The model under review builds one solid part; all positions refer to its coordinate system, in mm. Face numbers are marked on the shaded views. A direction names the side the tool comes from. Coordinates: 2 decimals unless noted, no trailing zeros. Write each loop counter-clockwise with the first axis right and the second up, starting at its lowest first coordinate (ties: lowest second). Pieces come first, ordered by that corner, then holes. Notation, with made-up numbers: (-37.5, -25) - (1.5, -25) arc R19 cw to (1.5, -21) - close; hole circle Ø8 at (79, -20). An arc over 180 degrees is marked (long way). Put each result on its own line as item: value.
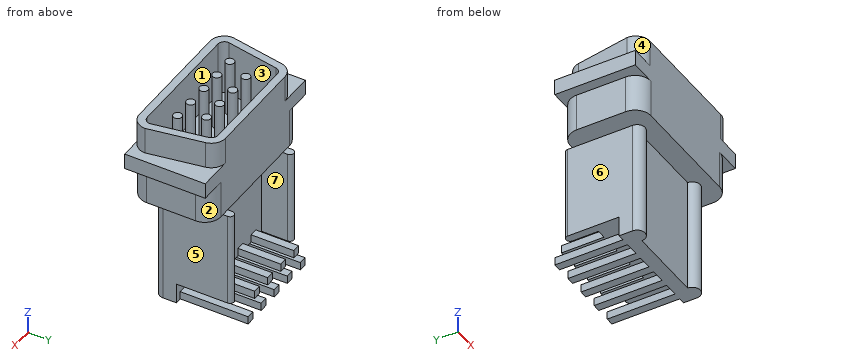
from build123d import *

# Parameters (mm, degrees)
SKETCH_1_W          = 21.2
SKETCH_1_H          = 10.2
EXTRUDE_1_DEPTH     = 2
EXTRUDE_2_DEPTH     = 3.4
EXTRUDE_3_DEPTH     = 4.8
EXTRUDE_4_DEPTH     = 12
EXTRUDE_5_DEPTH     = 2.6
SKETCH_6_R          = 0.545
CUT_EXTRUDE_1_DEPTH = 7
SKETCH_7_W          = 1
SKETCH_7_H          = 1
EXTRUDE_6_DEPTH     = 8.6
SKETCH_8_W          = 1
SKETCH_8_H          = 1
EXTRUDE_7_DEPTH     = 5.4


with BuildPart() as part:
    # Эскиз1 → Бобышка-Вытянуть1 (new body)
    with BuildSketch(Plane.XY):
        Rectangle(SKETCH_1_W, SKETCH_1_H)
    extrude(amount=EXTRUDE_1_DEPTH)

    # Эскиз2 → Бобышка-Вытянуть2 (add)
    with BuildSketch(Plane.XY.offset(2)):
        with BuildLine():
            Line((-6.3, 5.1), (6.3, 5.1))
            ThreePointArc((6.3, 5.1), (7.4561981, 4.679567307), (8.072281221, 3.614673282))
            Line((8.072281221, 3.614673282), (9.3, -3.3))
            ThreePointArc((9.3, -3.3), (8.772792206, -4.572792206), (7.5, -5.1))
            Line((7.5, -5.1), (-7.5, -5.1))
            ThreePointArc((-7.5, -5.1), (-8.772792206, -4.572792206), (-9.3, -3.3))
            Line((-9.3, -3.3), (-8.072281221, 3.614673282))
            ThreePointArc((-8.072281221, 3.614673282), (-7.4561981, 4.679567307), (-6.3, 5.1))
        make_face()
    extrude(amount=EXTRUDE_2_DEPTH)

    # Эскиз3 → Бобышка-Вытянуть3 (add)
    with BuildSketch(Plane(origin=(0, 0, 0), x_dir=(-1, 0, 0), z_dir=(0, 0, -1))):
        with BuildLine():
            Line((7.3, -5.1), (-7.3, -5.1))
            ThreePointArc((-7.3, -5.1), (-8.714213562, -4.514213562), (-9.3, -3.1))
            Line((-9.3, -3.1), (-9.3, 3.1))
            ThreePointArc((-9.3, 3.1), (-8.714213562, 4.514213562), (-7.3, 5.1))
            Line((-7.3, 5.1), (7.3, 5.1))
            ThreePointArc((7.3, 5.1), (8.714213562, 4.514213562), (9.3, 3.1))
            Line((9.3, 3.1), (9.3, -3.1))
            ThreePointArc((9.3, -3.1), (8.714213562, -4.514213562), (7.3, -5.1))
        make_face()
    extrude(amount=EXTRUDE_3_DEPTH)

    # Эскиз4 → Бобышка-Вытянуть4 (add)
    with BuildSketch(Plane(origin=(0, 0, -4.8), x_dir=(-1, 0, 0), z_dir=(0, 0, -1))):
        with BuildLine():
            Line((4.85, -2.5), (-4.85, -2.5))
            ThreePointArc((-4.85, -2.5), (-5.85, -3.5), (-6.85, -2.5))
            Line((-6.85, -2.5), (-6.85, 5.7))
            ThreePointArc((-6.85, 5.7), (-6.35, 6.2), (-5.85, 5.7))
            Line((-5.85, 5.7), (-5.85, 2.4))
            Line((-5.85, 2.4), (5.85, 2.4))
            Line((5.85, 2.4), (5.85, 5.7))
            ThreePointArc((5.85, 5.7), (6.35, 6.2), (6.85, 5.7))
            Line((6.85, 5.7), (6.85, -2.5))
            ThreePointArc((6.85, -2.5), (5.85, -3.5), (4.85, -2.5))
        make_face()
    extrude(amount=EXTRUDE_4_DEPTH)

    # Эскиз5 → Бобышка-Вытянуть5 (add)
    with BuildSketch(Plane(origin=(0, 0, -16.8), x_dir=(-1, 0, 0), z_dir=(0, 0, -1))):
        with BuildLine():
            Line((6.85, -0.8), (-6.85, -0.8))
            Line((-6.85, -0.8), (-6.85, -2.5))
            ThreePointArc((-6.85, -2.5), (-5.85, -3.5), (-4.85, -2.5))
            Line((-4.85, -2.5), (4.85, -2.5))
            ThreePointArc((4.85, -2.5), (5.85, -3.5), (6.85, -2.5))
            Line((6.85, -2.5), (6.85, -0.8))
        make_face()
    extrude(amount=EXTRUDE_5_DEPTH)

    # Эскиз6 → Вырез-Вытянуть1 (cut)
    with BuildSketch(Plane.XY.offset(5.4)):
        with BuildLine():
            Line((7.5, -4.1), (-7.5, -4.1))
            ThreePointArc((-7.5, -4.1), (-8.113141025, -3.813865822), (-8.287680543, -3.160145208))
            Line((-8.287680543, -3.160145208), (-7.114972471, 3.444700547))
            ThreePointArc((-7.114972471, 3.444700547), (-6.831670489, 3.934385426), (-6.3, 4.127718779))
            Line((-6.3, 4.127718779), (6.3, 4.127718779))
            ThreePointArc((6.3, 4.127718779), (6.831670489, 3.934385426), (7.114972471, 3.444700547))
            Line((7.114972471, 3.444700547), (8.287680543, -3.160145208))
            ThreePointArc((8.287680543, -3.160145208), (8.113141025, -3.813865822), (7.5, -4.1))
        make_face()
        with Locations((0, -1.42)):
            Circle(SKETCH_6_R, mode=Mode.SUBTRACT)
        with Locations((-2.77, -1.42)):
            Circle(SKETCH_6_R, mode=Mode.SUBTRACT)
        with Locations((-5.54, -1.42)):
            Circle(SKETCH_6_R, mode=Mode.SUBTRACT)
        with Locations((2.77, -1.42)):
            Circle(SKETCH_6_R, mode=Mode.SUBTRACT)
        with Locations((5.54, -1.42)):
            Circle(SKETCH_6_R, mode=Mode.SUBTRACT)
        with Locations((1.385, 1.42)):
            Circle(SKETCH_6_R, mode=Mode.SUBTRACT)
        with Locations((-1.385, 1.42)):
            Circle(SKETCH_6_R, mode=Mode.SUBTRACT)
        with Locations((-4.155, 1.42)):
            Circle(SKETCH_6_R, mode=Mode.SUBTRACT)
        with Locations((4.155, 1.42)):
            Circle(SKETCH_6_R, mode=Mode.SUBTRACT)
    extrude(amount=-CUT_EXTRUDE_1_DEPTH, mode=Mode.SUBTRACT)

    # Эскиз7 → Бобышка-Вытянуть6 (add)
    with BuildSketch(Plane(origin=(0, -0.8, 0), x_dir=(1, 0, 0), z_dir=(0, 1, 0))):
        with Locations((0, 18.9)):
            Rectangle(SKETCH_7_W, SKETCH_7_H)
        with Locations((2.77, 18.9)):
            Rectangle(SKETCH_7_W, SKETCH_7_H)
        with Locations((5.54, 18.9)):
            Rectangle(SKETCH_7_W, SKETCH_7_H)
        with Locations((-2.77, 18.9)):
            Rectangle(SKETCH_7_W, SKETCH_7_H)
        with Locations((-5.54, 18.9)):
            Rectangle(SKETCH_7_W, SKETCH_7_H)
    extrude(amount=EXTRUDE_6_DEPTH)

    # Эскиз8 → Бобышка-Вытянуть7 (add)
    with BuildSketch(Plane(origin=(0, 2.4, 0), x_dir=(1, 0, 0), z_dir=(0, 1, 0))):
        with Locations((-1.385, 16.3)):
            Rectangle(SKETCH_8_W, SKETCH_8_H)
        with Locations((1.385, 16.3)):
            Rectangle(SKETCH_8_W, SKETCH_8_H)
        with Locations((4.155, 16.3)):
            Rectangle(SKETCH_8_W, SKETCH_8_H)
        with Locations((-4.155, 16.3)):
            Rectangle(SKETCH_8_W, SKETCH_8_H)
    extrude(amount=EXTRUDE_7_DEPTH)


solid = part.part
1. Consider section A-A on z = -10.5. State the section outline as (x, y) points.
Determined:
outline: (-6.85, -2.5) arc R1 ccw to (-4.85, -2.5) - (4.85, -2.5) arc R1 ccw to (6.85, -2.5) - (6.85, 5.7) arc R0.5 ccw to (5.85, 5.7) - (5.85, 2.4) - (-5.85, 2.4) - (-5.85, 5.7) arc R0.5 ccw to (-6.85, 5.7) - close
2. Machinability: for the marked faces 5, 6 and 7, which of the approach directions +Z, -Z, +X, -X, +Y, -Y give a long, thin tool a straight path to every point of the face, cutting with its end or side? Answer none if there is none.
Determined:
face 5: -Z, +X, +Y, -Y
face 6: -Z, -X, +Y, -Y
face 7: +Y
3. Consider section D-D on x = 5.54. State the section outline as (y, z) points (3 decimals), plus the area to 3 significant figures.
Determined:
outline: (-5.1, -4.8) - (-3.451, -4.8) - (-3.451, -19.4) - (7.8, -19.4) - (7.8, -18.4) - (-0.8, -18.4) - (-0.8, -16.8) - (2.4, -16.8) - (2.4, -4.8) - (5.1, -4.8) - (5.1, 5.4) - (4.128, 5.4) - (4.128, -1.6) - (-0.875, -1.6) - (-0.875, 5.4) - (-1.965, 5.4) - (-1.965, -1.6) - (-4.1, -1.6) - (-4.1, 5.4) - (-5.1, 5.4) - close
area: 140 mm^2
4. The part is to be moulded in two halves that separate along Y. For the marked faces 1, 2, 3 and 4, say which applies: +Y half, -Y half, draft (parallel to the pull), parting line (faces both ways), or undercut.
Determined:
face 1: undercut
face 2: +Y half
face 3: undercut
face 4: -Y half
5. To check wall thickness, follow probe 1 along X at (y, z) = (5.5, -5); probe 2 along Z at (x, y) = (1, 4.25); probe 3 along Z at (x, y) = (-0.25, 1.75). State the ranges of each line that lie inside material, in increasing order.
Determined:
probe 1: x = -6.85 to -5.85, 5.85 to 6.85
probe 2: z = -16.8 to -15.8, -4.8 to 5.4
probe 3: z = -19.4 to -18.4, -16.8 to -1.6
6. Consider section B-B on x = 2.77. State the section outline as (y, z) points (3 decimals), plus the area to 3 significant figures.
Determined:
outline: (-5.1, -4.8) - (-2.5, -4.8) - (-2.5, -19.4) - (7.8, -19.4) - (7.8, -18.4) - (-0.8, -18.4) - (-0.8, -16.8) - (2.4, -16.8) - (2.4, -4.8) - (5.1, -4.8) - (5.1, 5.4) - (4.128, 5.4) - (4.128, -1.6) - (-0.875, -1.6) - (-0.875, 5.4) - (-1.965, 5.4) - (-1.965, -1.6) - (-4.1, -1.6) - (-4.1, 5.4) - (-5.1, 5.4) - close
area: 126 mm^2
7. For pin 1 Ø0.8 at (y, z) = (4, -16.5) entering from +X; pin 2 Ø8 at (x, z) = (6, -7.5) entering from +Y; pin 3 Ø2 at (y, z) = (-2.5, -1.5) entering from -X, all flat-tipped, find the tip position at first contact; note any pin that passes through.
Determined:
pin 1: stops at x = 6.85
pin 2: stops at y = 6.2
pin 3: stops at x = -9.3
8. Consider section C-C on z = -4. State the section outline as (x, y) points, plus the area to 3 significant figures.
Determined:
outline: (-9.3, -3.1) arc R2 ccw to (-7.3, -5.1) - (7.3, -5.1) arc R2 ccw to (9.3, -3.1) - (9.3, 3.1) arc R2 ccw to (7.3, 5.1) - (-7.3, 5.1) arc R2 ccw to (-9.3, 3.1) - close
area: 186 mm^2
